from build123d import *

# Parameters (mm, degrees)
F1_DEPTH = 215.9
F2_W     = 57.15
F2_H     = 209.55
F3_DEPTH = 32.5744088888
F4_R     = 3.175
F5_DEPTH = 81.281


# Not quite as in the source:
# - a feature names something its author has since deleted; it is built from what else it names


with BuildPart() as f1:
    # F0 (on Front) → F1 (new body)
    with BuildSketch(Plane.XZ):
        with BuildLine():
            Line((-36.83, 0), (-30.48, 0))
            ThreePointArc((-30.48, 0), (0, 30.48), (30.48, 0))
            Line((30.48, 0), (36.83, 0))
            Line((36.83, 0), (49.53, 0))
            Line((49.53, 0), (49.53, 6.35))
            Line((49.53, 6.35), (36.278456417, 6.35))
            ThreePointArc((36.278456417, 6.35), (34.5670828322, 12.7108490854), (31.75, 18.66511184))
            ThreePointArc((31.75, 18.66511184), (30.2489666674, 21.0106857469), (28.575, 23.2361415687))
            ThreePointArc((28.575, 23.2361415687), (0, 36.83), (-28.575, 23.2361415687))
            ThreePointArc((-28.575, 23.2361415687), (-30.2489666674, 21.0106857469), (-31.75, 18.66511184))
            ThreePointArc((-31.75, 18.66511184), (-34.5670828322, 12.7108490854), (-36.278456417, 6.35))
            Line((-36.278456417, 6.35), (-49.53, 6.35))
            Line((-49.53, 6.35), (-49.53, 0))
            Line((-49.53, 0), (-36.83, 0))
        make_face()
        with BuildLine():
            ThreePointArc((28.575, 23.2361415687), (30.2489666674, 21.0106857469), (31.75, 18.66511184))
            Line((31.75, 18.66511184), (31.75, 43.18))
            Line((31.75, 43.18), (28.575, 43.18))
            Line((28.575, 43.18), (28.575, 23.2361415687))
        make_face()
        with BuildLine():
            Line((-28.575, 43.18), (-28.575, 23.2361415687))
            ThreePointArc((-28.575, 23.2361415687), (0, 36.83), (28.575, 23.2361415687))
            Line((28.575, 23.2361415687), (28.575, 43.18))
            Line((28.575, 43.18), (-28.575, 43.18))
        make_face()
        with BuildLine():
            Line((-31.75, 43.18), (-31.75, 18.66511184))
            ThreePointArc((-31.75, 18.66511184), (-30.2489666674, 21.0106857469), (-28.575, 23.2361415687))
            Line((-28.575, 23.2361415687), (-28.575, 43.18))
            Line((-28.575, 43.18), (-31.75, 43.18))
        make_face()
    extrude(amount=-F1_DEPTH)

    # F2 (on face) → F3 (cut, through all)
    with BuildSketch(Plane.XY.offset(43.18)):
        with Locations((0, 107.95)):
            Rectangle(F2_W, F2_H)
    extrude(amount=-F3_DEPTH, mode=Mode.SUBTRACT)

    # F4 (on face) → F5 (cut, through all)
    with BuildSketch(Plane.YZ.offset(31.75)):
        with Locations((12.7, 30.92255592)):
            Circle(F4_R)
        with Locations((25.4, 30.92255592)):
            Circle(F4_R)
        with Locations((38.1, 30.92255592)):
            Circle(F4_R)
        with Locations((50.8, 30.92255592)):
            Circle(F4_R)
        with Locations((63.5, 30.92255592)):
            Circle(F4_R)
        with Locations((152.4, 30.92255592)):
            Circle(F4_R)
        with Locations((165.1, 30.92255592)):
            Circle(F4_R)
        with Locations((177.8, 30.92255592)):
            Circle(F4_R)
        with Locations((190.5, 30.92255592)):
            Circle(F4_R)
        with Locations((203.2, 30.92255592)):
            Circle(F4_R)
    extrude(amount=-F5_DEPTH, mode=Mode.SUBTRACT)


solid = f1.part
For this review, take the finished solid that the model builds, in its own axes (mm). A direction names the side the tool comes from. Round coordinates to 2 decimals unless told otherwise and drop trailing zeros. Write each loop counter-clockwise with the first axis right and the second up, starting at its lowest first coordinate (ties: lowest second). Pieces come first, ordered by that corner, then holes. Notation, with made-up numbers: M 24,-9.75 L 77,-9.75 A15 cw 77,-5.75 Z; hole C 86,59 d11. An arc over 180 degrees is marked long. Write item = value, one per line. Start each with the question number.
(1) The part is to be moulded in two halves that separate along Y. For faces 1 (the face through (30.185, 187.328, 31.062)), 2 (the face through (31, 107, 43.18)), say which applies: +Y half, -Y half, draft (parallel to the pull), parting line (faces both ways), or undercut.
(2) For faces 3 (the face through (-28.575, 106, 27)), 4 (the face through (-30.14, 180.733, 29.707)), 5 (the face through (43, 106, 6.35)), list the 3-axis set-ups (+Z, -Z, +X, -X, +Y, -Y) from which the entire face can be reached by the end or side of a thin tool; tool diameter is ignored.
(3) For line 1 along X through (y, z) = (204, 36) (3 decimals); line 2 along Z through (x, y) = (-30.6, 203.2); line 3 along Y through (x, z) = (-3.5, 38.5) (3 decimals), list the stretches that pass through material, from the lowest coordinate up.
(4) We need section D-D (z = 25). Give the boundary of the cut face in (x, y) (3 decimals), then the cut area to 3 significant figures.
(5) Clearance check with flat-ended pins moving along their axes: pin 1 Ø4 at (y, z) = (134, 36.5) entering from -X; pin 2 Ø8.5 at (y, z) = (152.4, 30.92) entering from +X; pin 3 Ø4 at (y, z) = (25.4, 30.92) entering from -X; pin 4 Ø4 at (x, y) = (43.5, 66.5) entering from +Z. State where each tip first meets the part, or that it passes through.
(6) We need section C-C (x = 0). Give the boundary of the cut face in (y, z) (3 decimals).
(7) We need section A-A (y = 63.5). Give the boundary of the cut face in (x, z) (3 decimals), then the cut area to 3 significant figures.
(8) We need section B-B (y = 18). Give the boundary of the cut face in (x, z) (3 decimals), then the cut area to 3 significant figures.
Results found:
q1.face_1 = undercut
q1.face_2 = draft
q2.face_3 = +Z, -Z
q2.face_4 = +X, -X
q2.face_5 = +Z, +X, +Y, -Y
q3.line_1 = -31.75 to -28.575, 28.575 to 31.75
q3.line_2 = 0 to 27.75, 34.1 to 43.18
q3.line_3 = 0 to 3.175, 212.725 to 215.9
q4.outline = M -31.75,0 L -17.436,0 L -17.436,3.175 L -28.575,3.175 L -28.575,212.725 L -17.436,212.725 L -17.436,215.9 L -31.75,215.9 Z; M 17.436,0 L 31.75,0 L 31.75,215.9 L 17.436,215.9 L 17.436,212.725 L 28.575,212.725 L 28.575,3.175 L 17.436,3.175 Z
q4.area = 1,510 mm²
q5.pin_1 = -31.75
q5.pin_2 = 31.75
q5.pin_3 = through
q5.pin_4 = 6.35
q6.outline = M 0,30.48 L 3.175,30.48 L 3.175,43.18 L 0,43.18 Z; M 212.725,30.48 L 215.9,30.48 L 215.9,43.18 L 212.725,43.18 Z
q7.outline = M -49.53,0 L -30.48,0 A30.48 cw -28.575,10.607 L -28.575,27.748 L -31.75,27.748 L -31.75,18.665 A36.83 ccw -36.278,6.35 L -49.53,6.35 Z; M -31.75,34.098 L -28.575,34.098 L -28.575,43.18 L -31.75,43.18 Z; M 28.575,10.607 A30.48 cw 30.48,0 L 49.53,0 L 49.53,6.35 L 36.278,6.35 A36.83 ccw 31.75,18.665 L 31.75,27.748 L 28.575,27.748 Z; M 28.575,34.098 L 31.75,34.098 L 31.75,43.18 L 28.575,43.18 Z
q7.area = 499 mm²
q8.outline = M -49.53,0 L -30.48,0 A30.48 cw -28.575,10.607 L -28.575,43.18 L -31.75,43.18 L -31.75,18.665 A36.83 ccw -36.278,6.35 L -49.53,6.35 Z; M 28.575,10.607 A30.48 cw 30.48,0 L 49.53,0 L 49.53,6.35 L 36.278,6.35 A36.83 ccw 31.75,18.665 L 31.75,43.18 L 28.575,43.18 Z
q8.area = 539 mm²
